from build123d import *

# Parameters (mm, degrees)
BOSS_EXTRUDE1_DEPTH  = 19.05
CUT_SWEEP1_PROFILE_R = 6.35
FILLET1_R            = 30
FILLET2_R            = 20
SKETCH10_W           = 5
SKETCH10_H           = 15
SKETCH10_W_2         = 15
SKETCH10_H_2         = 5
BOSS_EXTRUDE2_DEPTH  = 10
FILLET3_R            = 1
BOSS_EXTRUDE3_DEPTH  = 19.05
SKETCH14_W           = 12
SKETCH14_H           = 10
CUT_EXTRUDE1_DEPTH   = 39


with BuildPart() as part:
    # Sketch1 → Boss-Extrude1 (new body)
    with BuildSketch(Plane.XY):
        Polygon((-100, 0), (0, 0), (0, 250), (65, 250), (65, 211.9), (38.1, 211.9), (38.1, -38.1), (-100, -38.1), align=None)
    extrude(amount=BOSS_EXTRUDE1_DEPTH)

    # Cut-Sweep1: sweep along a path in Sketch2
    with BuildLine(Plane(origin=(0, 0, 0), x_dir=(-1, 0, 0), z_dir=(0, 0, -1))) as cut_sweep1_path:
        Line((-65, 230.95), (-39.05, 230.95))
        ThreePointArc((-39.05, 230.95), (-24.907864376, 225.092135624), (-19.05, 210.95))
        Line((-19.05, 210.95), (-19.05, 0.95))
        ThreePointArc((-19.05, 0.95), (-13.192135624, -13.192135624), (0.95, -19.05))
        Line((0.95, -19.05), (100, -19.05))
    # Cut-Sweep1 profile (on start of the path) → Cut-Sweep1 (sweep, cut)
    with BuildSketch(Plane(origin=(65, 230.95, 0), x_dir=(0, 0, -1), z_dir=(-1, 0, 0))):
        Circle(CUT_SWEEP1_PROFILE_R)
    sweep(path=cut_sweep1_path.line, mode=Mode.SUBTRACT)

    # Fillet1
    fillet1_edges = [part.edges().sort_by_distance(p)[0] for p in [
        (0, 250, 9.525),
        (38.1, -38.1, 9.525),
    ]]
    fillet(fillet1_edges, radius=FILLET1_R)

    # Fillet2
    fillet2_edges = [part.edges().sort_by_distance(p)[0] for p in [
        (0, 0, 9.525),
    ]]
    fillet(fillet2_edges, radius=FILLET2_R)

    # Sketch10 → Boss-Extrude2 (add)
    with BuildSketch(Plane(origin=(0, 0, 0), x_dir=(-1, 0, 0), z_dir=(0, 0, -1))):
        with Locations((-6.35, 120)):
            Rectangle(SKETCH10_W, SKETCH10_H)
        with Locations((-31.75, 120)):
            Rectangle(SKETCH10_W, SKETCH10_H)
        with Locations((60, -6.35)):
            Rectangle(SKETCH10_W_2, SKETCH10_H_2)
        with Locations((60, -31.75)):
            Rectangle(SKETCH10_W_2, SKETCH10_H_2)
    extrude(amount=BOSS_EXTRUDE2_DEPTH)

    # Fillet3
    fillet3_edges = [part.edges().sort_by_distance(p)[0] for p in [
        (-67.5, -31.75, 0),
        (-60, -29.25, 0),
        (-52.5, -31.75, 0),
        (-60, -34.25, 0),
        (8.85, 120, 0),
        (6.35, 112.5, 0),
        (3.85, 120, 0),
        (6.35, 127.5, 0),
        (-52.5, -6.35, 0),
        (-60, -8.85, 0),
        (-67.5, -6.35, 0),
        (-60, -3.85, 0),
        (34.25, 120, 0),
        (31.75, 112.5, 0),
        (29.25, 120, 0),
        (31.75, 127.5, 0),
    ]]
    fillet(fillet3_edges, radius=FILLET3_R)

    # Sketch13 → Boss-Extrude3 (add)
    with BuildSketch(Plane.XY.offset(19.05)):
        Polygon((55, 221.425), (43, 221.425), (43, 211.425), (51, 211.425), (51, 189.425), (41, 189.425), (41, 171.425), (36.549895251, 171.425), (36.549895251, 223.572995821), (65, 223.572995821), (65, 211.9), (65, 211.425), (55, 211.425), align=None)
    extrude(amount=-BOSS_EXTRUDE3_DEPTH)

    # Sketch14 → Cut-Extrude1 (cut)
    with BuildSketch(Plane.XY.offset(19.05)):
        with Locations((49, 216.42)):
            Rectangle(SKETCH14_W, SKETCH14_H)
    extrude(amount=-CUT_EXTRUDE1_DEPTH, mode=Mode.SUBTRACT)


solid = part.part
Geometry: final body of the model. Coordinates: model frame, mm. A direction names the side the tool comes from. Coordinates: 2 decimals unless noted, no trailing zeros. Order: outer loops, then holes, each group sorted by start corner. A loop starts at its lowest first (then second) coordinate and runs counter-clockwise, first axis right, second up. Notation, with made-up numbers: M 75,56.25 L 109,56.25 A25 cw 109,77.25 Z; hole C 2.25,-27.5 d1. An arc over 180 degrees is marked long. One line per question, with ' | ' between items. Start each with the question number.
Item 1: Cut plane B-B, the plane x = -35. Return the cut outline in (y, z), then the cut area to 3 significant figures.
Item 2: Pin query (flat end, axial travel): pin 1 Ø4.5 at (y, z) = (123.5, -5) entering from +X; pin 2 Ø2 at (x, z) = (36, 3.5) entering from -Y; pin 3 Ø12 at (x, z) = (-67, -3.5) entering from -Y; pin 4 Ø3 at (x, z) = (48.5, 11.5) entering from -Y (3 decimals). Return the tip coordinate at first contact, or that it passes through.
Item 3: Cut plane C-C, the plane z = 12. Return the cut outline in (x, y) (3 decimals).
Item 4: Ray query, probe 1 along Y at (x, z) = (-55, -2.5); probe 2 along X at (y, z) = (133.5, 13.5); probe 3 along Y at (x, z) = (-43, 13.5). Return the intervals inside material, ascending. Write a range as [from, to].
Item 5: Set-up query: faces 1 (the flat face through (29.25, 120, -5)), 2 (the flat face through (49, 221.42, 10)), 3 (the flat face through (0, 119, 9)). Return all of +Z, -Z, +X, -X, +Y, -Y with unobstructed straight access to the full face (end or side cutting, diameter ignored); none if empty.
Item 6: Cut plane A-A, the plane y = 123. Return the cut outline in (x, z), then the cut area to 3 significant figures.
Item 7: Cut plane D-D, the plane x = -57.5. Return the cut outline in (y, z).
A:
1) outline: M -38.1,0 L -25.4,0 A6.35 cw -12.7,0 L 0,0 L 0,19.05 L -38.1,19.05 Z | area: 662 mm2
2) pin 1: stops at x = 34.25 | pin 2: stops at y = -21.38 | pin 3: stops at y = -38.1 | pin 4: stops at y = 189.425
3) outline: M -100,-38.1 L 8.1,-38.1 A30 ccw 38.1,-8.1 L 38.1,171.425 L 41,171.425 L 41,189.425 L 51,189.425 L 51,211.42 L 43,211.42 L 43,221.42 L 55,221.42 L 55,211.425 L 65,211.425 L 65,250 L 30,250 A30 ccw 0,220 L 0,20 A20 cw -20,0 L -100,0 Z
4) probe 1: y = [-34.25, -29.25], [-8.85, -3.85] | probe 2: x = [0, 38.1] | probe 3: y = [-38.1, 0]
5) face 1: -Z, +Y, -Y | face 2: +Z, -Z | face 3: +Z, -Z, -X, +Y
6) outline: M 0,0 L 2.85,0 A1 cw 3.85,-1 L 3.85,-10 L 8.85,-10 L 8.85,-1 A1 cw 9.85,0 L 12.7,0 A6.35 cw 25.4,0 L 28.25,0 A1 cw 29.25,-1 L 29.25,-10 L 34.25,-10 L 34.25,-1 A1 cw 35.25,0 L 38.1,0 L 38.1,19.05 L 0,19.05 Z | area: 763 mm2
7) outline: M -38.1,0 L -35.25,0 A1 cw -34.25,-1 L -34.25,-10 L -29.25,-10 L -29.25,-1 A1 cw -28.25,0 L -25.4,0 A6.35 cw -12.7,0 L -9.85,0 A1 cw -8.85,-1 L -8.85,-10 L -3.85,-10 L -3.85,-1 A1 cw -2.85,0 L 0,0 L 0,19.05 L -38.1,19.05 Z
